from build123d import *

# Parameters (mm, degrees)
SKETCH1_R           = 13.97
BOSS_EXTRUDE1_DEPTH = 3.175
SKETCH2_W           = 3.175
SKETCH2_H           = 53.34
BOSS_EXTRUDE2_DEPTH = 25.4
CUT_EXTRUDE1_DEPTH  = 51.927
FILLET1_R           = 1.5875
FILLET2_R           = 3.175
FILLET3_R           = 3.175


with BuildPart() as part:
    # Sketch1 → Boss-Extrude1 (new body)
    with BuildSketch(Plane(origin=(0, 0, 0), x_dir=(1, 0, 0), z_dir=(0, 1, 0))):
        with BuildLine():
            ThreePointArc((4.499810369, -18.772216775), (19.304, 0), (4.499810369, 18.772216775))
            Line((4.499810369, 18.772216775), (-28.448, 26.67))
            Line((-28.448, 26.67), (-31.623, 26.67))
            Line((-31.623, 26.67), (-31.623, -26.67))
            Line((-31.623, -26.67), (-28.448, -26.67))
            Line((-28.448, -26.67), (4.499810369, -18.772216775))
        make_face()
        Circle(SKETCH1_R, mode=Mode.SUBTRACT)
    extrude(amount=BOSS_EXTRUDE1_DEPTH)

    # Sketch2 → Boss-Extrude2 (add)
    with BuildSketch(Plane(origin=(0, 3.175, 0), x_dir=(1, 0, 0), z_dir=(0, 1, 0))):
        with Locations((-30.0355, 0)):
            Rectangle(SKETCH2_W, SKETCH2_H)
    extrude(amount=BOSS_EXTRUDE2_DEPTH)

    # Sketch6 → Cut-Extrude1 (cut, through all)
    with BuildSketch(Plane.ZY.offset(31.623)):
        with BuildLine():
            Line((-20.32, 11.1125), (-20.32, 14.2875))
            Line((-20.32, 14.2875), (-20.32, 17.4625))
            ThreePointArc((-20.32, 17.4625), (-23.495, 14.2875), (-20.32, 11.1125))
        make_face()
        with BuildLine():
            ThreePointArc((-20.32, 11.1125), (-18.07493597, 12.04243597), (-17.145, 14.2875))
            Line((-17.145, 14.2875), (-20.32, 14.2875))
            Line((-20.32, 14.2875), (-20.32, 11.1125))
        make_face()
        with BuildLine():
            Line((-20.32, 14.2875), (-17.145, 14.2875))
            ThreePointArc((-17.145, 14.2875), (-18.07493597, 16.53256403), (-20.32, 17.4625))
            Line((-20.32, 17.4625), (-20.32, 14.2875))
        make_face()
        with BuildLine():
            ThreePointArc((23.495, 14.2875), (20.32, 17.4625), (17.145, 14.2875))
            Line((17.145, 14.2875), (20.32, 14.2875))
            Line((20.32, 14.2875), (23.495, 14.2875))
        make_face()
        with BuildLine():
            Line((20.32, 14.2875), (17.145, 14.2875))
            ThreePointArc((17.145, 14.2875), (20.32, 11.1125), (23.495, 14.2875))
            Line((23.495, 14.2875), (20.32, 14.2875))
        make_face()
    extrude(amount=-CUT_EXTRUDE1_DEPTH, mode=Mode.SUBTRACT)

    # Fillet1
    fillet1_edges = [part.edges().sort_by_distance(p)[0] for p in [
        (-28.448, 3.175, 0),
    ]]
    fillet(fillet1_edges, radius=FILLET1_R)

    # Fillet2
    fillet2_edges = [part.edges().sort_by_distance(p)[0] for p in [
        (-31.623, 0, 0),
    ]]
    fillet(fillet2_edges, radius=FILLET2_R)

    # Fillet3
    fillet3_edges = [part.edges().sort_by_distance(p)[0] for p in [
        (-30.0355, 28.575, -26.67),
        (-30.0355, 28.575, 26.67),
    ]]
    fillet(fillet3_edges, radius=FILLET3_R)


solid = part.part
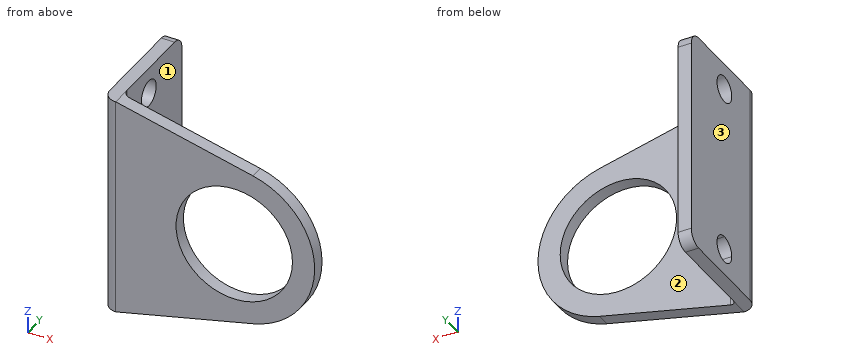
Verification items for the finished model (mm, model axes). Face numbers are marked on the shaded views. Give positions to 0.01 mm unless a question says otherwise; leave off trailing zeros. Order: outer loops, then holes, each group sorted by start corner. A loop starts at its lowest first (then second) coordinate and runs counter-clockwise, first axis right, second up. Notation, with made-up numbers: M 57,-39 L 115,-39 A19 cw 115,-14 Z; hole C 83,56.5 d9. An arc over 180 degrees is marked long. Answer as a JSON object with one key per item and string values. Group by question number.
1) Scan lines: line 1 along X through (y, z) = (20.5, 2.5); line 2 along Z through (x, y) = (0, 2); line 3 along Y through (x, z) = (13, 9.5) (3 decimals). Record each from-to range of solid material in increasing order. Write a range as [from, to].
2) Mould release check, pull along X, two halves, no side actions. Record for the marked faces 1, 2 and 3: released by +X, released by -X, zero draft, split by the parting line, or undercut.
3) Cross-section at D-D (y = 6.5). Enter the section's corners in (x, z), then the cut area to 3 significant figures.
4) Cross-section at C-C (y = 16.5). Enter the section's corners in (x, z), then the cut area to 3 significant figures.
5) Cross-section at B-B (x = 8.5). Enter the section's corners in (y, z) (3 decimals).
6) Depth check by flat-ended pin: pin 1 Ø8 at (x, z) = (1, -10.5) entering from +Y (3 decimals); pin 2 Ø1.5 at (x, y) = (1.5, 3) entering from +Z; pin 3 Ø2 at (x, y) = (8, 4.5) entering from +Z; pin 4 Ø4 at (y, z) = (5, 3) entering from +X. Enter the tip coordinate at first touch or a pass-through.
Result sheet:
{
 "1": {"line 1": "x = [-31.62, -28.45]", "line 2": "z = [-19.85, -13.97], [13.97, 19.85]", "line 3": "y = [0, 3.175]"},
 "2": {"face 1": "released by +X", "face 2": "zero draft", "face 3": "released by -X"},
 "3": {"outline": "M -31.62,-26.67 L -28.45,-26.67 L -28.45,26.67 L -31.62,26.67 Z", "area": "169 mm2"},
 "4": {"outline": "M -31.62,-26.67 L -28.45,-26.67 L -28.45,-22.6 L -31.62,-22.6 Z; M -31.62,-18.04 L -28.45,-18.04 L -28.45,18.04 L -31.62,18.04 Z; M -31.62,22.6 L -28.45,22.6 L -28.45,26.67 L -31.62,26.67 Z", "area": "140 mm2"},
 "5": {"outline": "M 0,-17.332 L 3.175,-17.332 L 3.175,-11.087 L 0,-11.087 Z; M 0,11.087 L 3.175,11.087 L 3.175,17.332 L 0,17.332 Z"},
 "6": {"pin 1": "stops at y = 3.175", "pin 2": "stops at z = 19.67", "pin 3": "passes through", "pin 4": "stops at x = 19.18"}
}
